CAD build for the part. Positions are in the model's coordinates, mm. A direction names the side the tool comes from. Round coordinates to 2 decimals unless told otherwise and drop trailing zeros. Loops run counter-clockwise (first coordinate to the right, second up) from the corner with the lowest first, then second, coordinate; pieces in that order, holes last.
```python
from build123d import *

# Parameters (mm, degrees)
F0_R     = 71.9118919296
F1_DEPTH = 25
F3_DEPTH = 50
F4_R     = 5
F5_R     = 5
F6_R     = 5
F7_R     = 5
F8_R     = 5


with BuildPart() as f1:
    # F0 (on Top) → F1 (new body)
    with BuildSketch(Plane.XY):
        Circle(F0_R)
    extrude(amount=F1_DEPTH)

    # F2 (on Front) → F3 (join, symmetric)
    with BuildSketch(Plane.XZ):
        Polygon((-34.6600189805, 43.438449502), (-36.7943756282, 42.5470620394), (-36.7943756282, -38.3929647505), (44.6020886302, -38.3929647505), align=None)
    extrude(amount=F3_DEPTH, both=True)

    # F4
    f4_edges = [f1.edges().sort_by_distance(p)[0] for p in [
        (44.602089, 0, -38.392965),
    ]]
    fillet(f4_edges, radius=F4_R)

    # F5
    f5_edges = [f1.edges().sort_by_distance(p)[0] for p in [
        (-36.794376, 0, -38.392965),
    ]]
    fillet(f5_edges, radius=F5_R)

    # F6
    f6_edges = [f1.edges().sort_by_distance(p)[0] for p in [
        (-71.911892, 0, 25),
    ]]
    fillet(f6_edges, radius=F6_R)

    # F7
    f7_edges = [f1.edges().sort_by_distance(p)[0] for p in [
        (-71.911892, 0, 0),
    ]]
    fillet(f7_edges, radius=F7_R)

    # F8
    f8_edges = [f1.edges().sort_by_distance(p)[0] for p in [
        (-16.800492, 0, 25),
    ]]
    fillet(f8_edges, radius=F8_R)


solid = f1.part
```
Item 1: Cut at D-D, the plane z = -27.5. Give the cut face in (x, y), plus the area to 3 significant figures.
Answers follow:
outline: (-36.79, -50) - (34.05, -50) - (34.05, 50) - (-36.79, 50) - close
area: 7,080 mm2
Item 2: Flat gauge pins, fed straight in: P1, Ø6, axis at x = -29, y = 9.5, coming from the +Z side; P2, Ø19, axis at x = -7.5, z = -18.5, coming from the -Y side; P3, Ø6, axis at x = -19.5, y = 27.5, coming from the +Z side. Where does each tip first touch, or does it go through?
Answers follow:
P1: stops at z = 40.69
P2: stops at y = -50
P3: stops at z = 30.88
Item 3: 3-axis set-ups, long thin cutter, end or side, ignore diameter. For faces 5 (the flat face through (-36.794, -1, -16)), 6 (the flat face through (-36.794, -1, 34)), 7 (the flat face through (-8, 50, -19)): which of +Z, -Z, +X, -X, +Y, -Y reach the whole face in a straight line?
Answers follow:
face 5: -Z, -X, +Y, -Y
face 6: +Z, -X, +Y, -Y
face 7: -Z, +X, -X, +Y
Item 4: Two-plate mould, pull along Z, no slides. Class faces 1 (the flat face through (22.105, -0.7, -15.167)), 2 (the flat face through (-26.35, -0.7, 34.86)), 3 (the cylindrical face through (-35.29, -0.7, -36.97)), 4 (the flat face through (-31, -50, 32)): released by +Z, released by -Z, zero draft, split by the parting line, or undercut.
Answers follow:
face 1: undercut
face 2: released by +Z
face 3: released by -Z
face 4: zero draft
Item 5: Cut at B-B, the plane x = 0. Give the cut face in (y, z), plus the area to 3 significant figures.
Answers follow:
outline: (-71.91, 5) arc R5 ccw to (-66.91, 0) - (-50, 0) - (-50, -38.39) - (50, -38.39) - (50, 0) - (66.91, 0) arc R5 ccw to (71.91, 5) - (71.91, 20) arc R5 ccw to (66.91, 25) - (-66.91, 25) arc R5 ccw to (-71.91, 20) - close
area: 7,410 mm2
Item 6: Probe line 1 (Y direction, x = -28, z = 33); line 2 (X direction, y = -32.5, z = -33); line 3 (Z direction, x = -56, y = 25). List the from-to ranges inside material, lowest first.
Answers follow:
line 1: y = -50 to 50
line 2: x = -36.79 to 37.78
line 3: z = 0 to 25
Item 7: Cut at C-C, the plane z = 9. Give the cut face in (x, y), plus the area to 3 significant figures.
Answers follow:
outline: circle Ø143.82 at (0, 0)
area: 16,200 mm2
Item 8: Cut at A-A, the plane y = 0. Give the cut face in (x, z).
Answers follow:
outline: (-71.91, 5) arc R5 ccw to (-66.91, 0) - (-36.79, 0) - (-36.79, -33.39) arc R5 ccw to (-31.79, -38.39) - (32.8, -38.39) arc R5 ccw to (36.39, -29.91) - (7.41, 0) - (66.91, 0) arc R5 ccw to (71.91, 5) - (71.91, 20) arc R5 ccw to (66.91, 25) - (-14.68, 25) arc R5 cw to (-18.27, 26.52) - (-34.66, 43.44) - (-36.79, 42.55) - (-36.79, 25) - (-66.91, 25) arc R5 ccw to (-71.91, 20) - close
